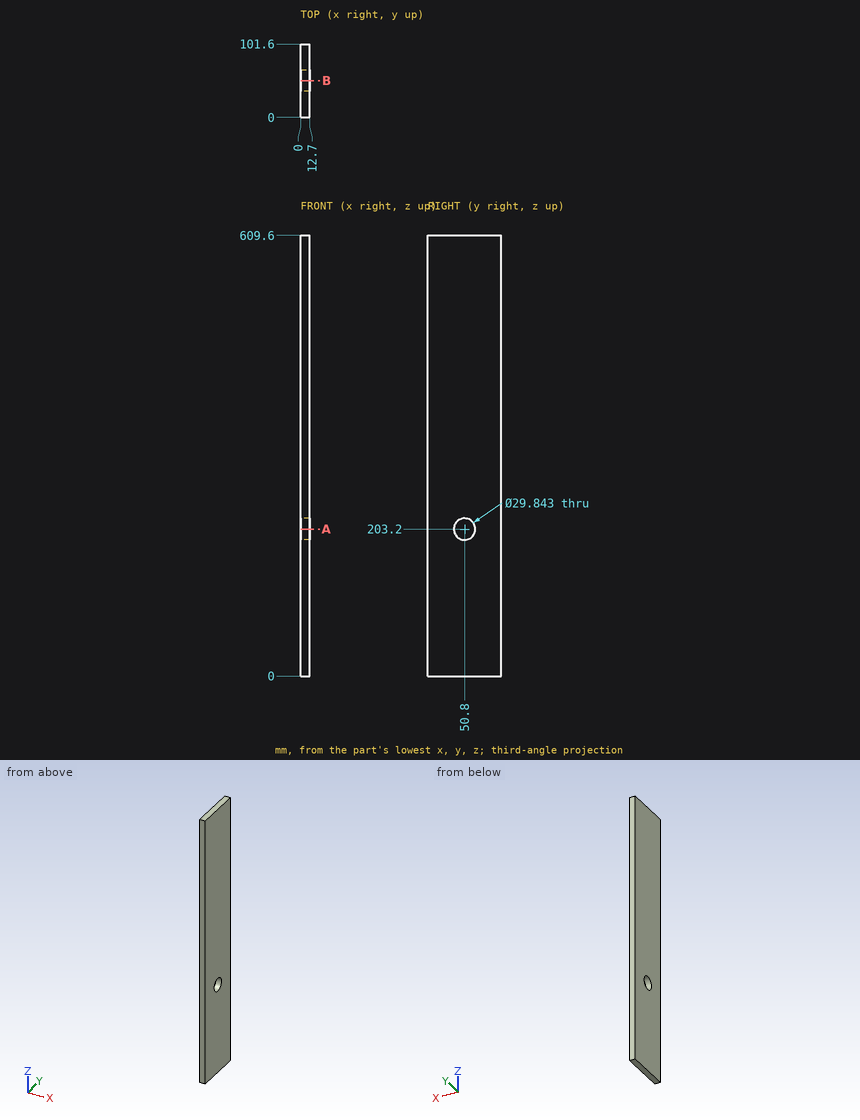
Part print with two shaded views. Sizes in mm from the minimum x, y, z corner. Round coordinates to 2 decimals unless told otherwise and drop trailing zeros. Order: outer loops, then holes, each group sorted by start corner. A loop starts at its lowest first (then second) coordinate and runs counter-clockwise, first axis right, second up. Notation, with made-up numbers: M -36,-36.5 L 17,-36.5 A32 ccw 17,-7.5 Z; hole C -4.5,-9.5 d10. An arc over 180 degrees is marked long. Use CSV: the item, a comma, the result in double quotes.
Item 1: Probe probe 1 along Z at (x, y) = (4.5, 50.8); probe 2 along Z at (x, y) = (12, 49). List the from-to ranges inside material, lowest first.
Worked answers:
probe 1,"0 to 188.28, 218.12 to 609.6"
probe 2,"0 to 188.39, 218.01 to 609.6"
Item 2: Saw through at A-A (z = 203.2). List the corners of the cut face in (x, y).
Worked answers:
outline,"M 0,0 L 12.7,0 L 12.7,35.88 L 0,35.88 Z; M 0,65.72 L 12.7,65.72 L 12.7,101.6 L 0,101.6 Z"
Item 3: Saw through at B-B (y = 50.8). List the corners of the cut face in (x, z), plus the area to 3 significant figures.
Worked answers:
outline,"M 0,0 L 12.7,0 L 12.7,188.28 L 0,188.28 Z; M 0,218.12 L 12.7,218.12 L 12.7,609.6 L 0,609.6 Z"
area,"7,360 mm²"
